Build history of the part. All positions in model axes, mm. A direction names the side the tool comes from. Give positions to 0.01 mm unless a question says otherwise; leave off trailing zeros. Loops run counter-clockwise (first coordinate to the right, second up) from the corner with the lowest first, then second, coordinate; pieces in that order, holes last. Notation, with made-up numbers: (-28.5, 54) -> (-3.5, 54) arc R9 cw to (-3.5, 65) -> close; hole circle Ø6 at (-29.5, 55.25). An arc over 180 degrees is marked (long way). Answer as a JSON object with one key per item and string values. Group by question number.
Q1. Wall check: probe 1 along X at (y, z) = (15.5, -38); probe 2 along Y at (x, z) = (0, -97) (3 decimals); probe 3 along X at (y, z) = (-5, -59). Give the ranges that are in metal, low to high. Write a range as from..to.
Q2. Band-saw the part on A-A, the plane x = 0. Write the cut outline in (y, z) (3 decimals), plus the area to 3 significant figures.
Q3. Two-plate mould, pull along Y, no slides. Class faces 4 (the flat face through (3, 3, 0)), 5 (the flat face through (0, -7.685, -148)), 6 (the cylindrical face through (-0.74, -3.32, -147.9)): pulls with the +Y half, pulls with the -Y half, needs draft (parallel to the pull), parting line crosses it, or undercut.
Q4. Band-saw the part on C-C, the plane z = -227. Count the separate pieces of the cut face and the enclosed holes in it, plus the area to 3 significant figures.
Q5. Drop flat-ended pins along their axis: pin 1 (7.5 mm diameter, centred on y = -1, z = -130.5, fed in from +X); pin 2 (0.7 mm diameter, centred on x = 18, z = -213, fed in from +Y); pin 3 (3.5 mm diameter, centred on x = 1, z = -81.5, fed in from +Y) (3 decimals). Give the stop position or say it passes through.
Q6. Tool access for faces 1 (the flat face through (0, 7.685, -148)), 2 (the flat face through (7.685, 0, -148)), 3 (the flat face through (-11.931, -14, -148)): list every direction of +Z, -Z, +X, -X, +Y, -Y with a clear straight run to the whole face (end or side of a thin tool).
Q7. Band-saw the part on B-B, the plane y = 0. Write the cut outline in (x, z) (3 decimals), plus the area to 3 significant figures.
from build123d import *

# Parameters (mm, degrees)
SKETCH1_R      = 3.4
EXTRUDE1_DEPTH = 300


with BuildPart() as part:
    # Sketch1 → Extrude1 (new body)
    with BuildSketch(Plane.XY):
        with BuildLine():
            Line((3.546734719, 7.685), (-3.215668941, 7.685))
            ThreePointArc((-3.215668941, 7.685), (-5.12166397, 8.084192802), (-6.707283616, 9.214671586))
            Line((-6.707283616, 9.214671586), (-9.994083925, 12.501471895))
            ThreePointArc((-9.994083925, 12.501471895), (-10.186794901, 12.789884252), (-10.254465997, 13.130089823))
            Line((-10.254465997, 13.130089823), (-10.254465997, 15.428464473))
            ThreePointArc((-10.254465997, 15.428464473), (-9.882491609, 16.326490085), (-8.984465997, 16.698464473))
            Line((-8.984465997, 16.698464473), (-6.775217878, 16.698464473))
            Line((-6.775217878, 16.698464473), (-6.775217878, 15.936))
            Line((-6.775217878, 15.936), (-5.6348, 15.936))
            ThreePointArc((-5.6348, 15.936), (-4.521248241, 16.397248241), (-4.06, 17.5108))
            Line((-4.06, 17.5108), (-4.06, 18.4252))
            ThreePointArc((-4.06, 18.4252), (-4.521248241, 19.538751759), (-5.6348, 20))
            Line((-5.6348, 20), (-13.0175, 20))
            Line((-13.0175, 20), (-16.825, 20))
            ThreePointArc((-16.825, 20), (-19.07006403, 19.07006403), (-20, 16.825))
            Line((-20, 16.825), (-20, -16.825))
            ThreePointArc((-20, -16.825), (-19.07006403, -19.07006403), (-16.825, -20))
            Line((-16.825, -20), (-13.0175, -20))
            Line((-13.0175, -20), (-5.6348, -20))
            ThreePointArc((-5.6348, -20), (-4.521248241, -19.538751759), (-4.06, -18.4252))
            Line((-4.06, -18.4252), (-4.06, -17.5108))
            ThreePointArc((-4.06, -17.5108), (-4.521248241, -16.397248241), (-5.6348, -15.936))
            Line((-5.6348, -15.936), (-6.775217878, -15.936))
            Line((-6.775217878, -15.936), (-6.775217878, -16.698464473))
            Line((-6.775217878, -16.698464473), (-8.984465997, -16.698464473))
            ThreePointArc((-8.984465997, -16.698464473), (-9.882491609, -16.326490085), (-10.254465997, -15.428464473))
            Line((-10.254465997, -15.428464473), (-10.254465997, -13.130554296))
            ThreePointArc((-10.254465997, -13.130554296), (-10.186794901, -12.790348725), (-9.994083925, -12.501936368))
            Line((-9.994083925, -12.501936368), (-6.707283616, -9.215136058))
            ThreePointArc((-6.707283616, -9.215136058), (-5.121525017, -8.084319577), (-3.21524064, -7.685))
            Line((-3.21524064, -7.685), (3.384844934, -7.685))
            ThreePointArc((3.384844934, -7.685), (5.234788394, -8.060064667), (6.792572846, -9.126025224))
            Line((6.792572846, -9.126025224), (9.994035567, -12.327487945))
            ThreePointArc((9.994035567, -12.327487945), (10.186746543, -12.615900302), (10.254417639, -12.956105874))
            Line((10.254417639, -12.956105874), (10.254417639, -15.439547173))
            ThreePointArc((10.254417639, -15.439547173), (9.878564697, -16.3303999), (8.984465997, -16.698464473))
            Line((8.984465997, -16.698464473), (6.775217878, -16.698464473))
            Line((6.775217878, -16.698464473), (6.775217878, -15.936))
            Line((6.775217878, -15.936), (5.6348, -15.936))
            ThreePointArc((5.6348, -15.936), (4.521248241, -16.397248241), (4.06, -17.5108))
            Line((4.06, -17.5108), (4.06, -18.4252))
            ThreePointArc((4.06, -18.4252), (4.521248241, -19.538751759), (5.6348, -20))
            Line((5.6348, -20), (13.34169248, -20))
            Line((13.34169248, -20), (17.15169248, -20))
            ThreePointArc((17.15169248, -20), (19.188402964, -18.962027535), (20, -16.825))
            Line((20, -16.825), (20, -13.015))
            Line((20, -13.015), (20, -5.5728))
            ThreePointArc((20, -5.5728), (19.517832289, -4.499539536), (18.426420946, -4.06))
            Line((18.426420946, -4.06), (17.5148, -4.06))
            ThreePointArc((17.5148, -4.06), (16.401248241, -4.521248241), (15.94, -5.6348))
            Line((15.94, -5.6348), (15.94, -6.775217878))
            Line((15.94, -6.775217878), (16.702464473, -6.775217878))
            Line((16.702464473, -6.775217878), (16.702464473, -8.984465997))
            ThreePointArc((16.702464473, -8.984465997), (16.363032482, -9.986041481), (15.382992443, -10.383394031))
            Line((15.382992443, -10.383394031), (13.085082266, -10.383394031))
            ThreePointArc((13.085082266, -10.383394031), (12.744876695, -10.315722936), (12.456464338, -10.12301196))
            Line((12.456464338, -10.12301196), (9.169664028, -6.83621165))
            ThreePointArc((9.169664028, -6.83621165), (8.107276575, -5.34917353), (7.685, -3.571075679))
            Line((7.685, -3.571075679), (7.685, 3.191327981))
            ThreePointArc((7.685, 3.191327981), (7.983205038, 5.049694415), (8.979790179, 6.646337802))
            Line((8.979790179, 6.646337802), (12.266590489, 9.933138111))
            ThreePointArc((12.266590489, 9.933138111), (12.592412986, 10.262627227), (13.039781689, 10.383394031))
            Line((13.039781689, 10.383394031), (15.37809843, 10.383394031))
            ThreePointArc((15.37809843, 10.383394031), (16.251511682, 10.035375209), (16.646241073, 9.182054333))
            Line((16.646241073, 9.182054333), (16.646241073, 6.972806215))
            Line((16.646241073, 6.972806215), (15.94, 6.972806215))
            Line((15.94, 6.972806215), (15.94, 5.832388337))
            ThreePointArc((15.94, 5.832388337), (16.321009151, 4.593446811), (17.502355238, 4.06))
            Line((17.502355238, 4.06), (18.4252, 4.06))
            ThreePointArc((18.4252, 4.06), (19.538751759, 4.521248241), (20, 5.6348))
            Line((20, 5.6348), (20, 13.01422635))
            Line((20, 13.01422635), (20, 16.82422635))
            ThreePointArc((20, 16.82422635), (19.070337634, 19.069790487), (16.825000094, 20))
            Line((16.825000094, 20), (13.290515583, 20))
            Line((13.290515583, 20), (5.6348, 20))
            ThreePointArc((5.6348, 20), (4.521248241, 19.538751759), (4.06, 18.4252))
            Line((4.06, 18.4252), (4.06, 17.5108))
            ThreePointArc((4.06, 17.5108), (4.521248241, 16.397248241), (5.6348, 15.936))
            Line((5.6348, 15.936), (6.775217878, 15.936))
            Line((6.775217878, 15.936), (6.775217878, 16.698464473))
            Line((6.775217878, 16.698464473), (8.984465997, 16.698464473))
            ThreePointArc((8.984465997, 16.698464473), (9.921702832, 16.349296475), (10.315534003, 15.429933551))
            Line((10.315534003, 15.429933551), (10.315534003, 13.130863473))
            ThreePointArc((10.315534003, 13.130863473), (10.284388293, 12.763467996), (10.106856362, 12.44030874))
            Line((10.106856362, 12.44030874), (6.825600792, 9.15905317))
            ThreePointArc((6.825600792, 9.15905317), (5.331011713, 8.099837434), (3.546734719, 7.685))
        make_face()
        Circle(SKETCH1_R, mode=Mode.SUBTRACT)
        with BuildLine():
            Line((11.904417639, 17.715), (11.904417639, 13.303394031))
            ThreePointArc((11.904417639, 13.303394031), (12.276392027, 12.405368419), (13.174417639, 12.033394031))
            Line((13.174417639, 12.033394031), (17.715, 12.033394031))
            ThreePointArc((17.715, 12.033394031), (18.164012806, 12.219381225), (18.35, 12.668394031))
            Line((18.35, 12.668394031), (18.35, 15.556))
            ThreePointArc((18.35, 15.556), (17.531656347, 17.531656347), (15.556, 18.35))
            Line((15.556, 18.35), (12.539417639, 18.35))
            ThreePointArc((12.539417639, 18.35), (12.090404833, 18.164012806), (11.904417639, 17.715))
        make_face(mode=Mode.SUBTRACT)
        with BuildLine():
            Line((-12.566039342, -18.35), (-15.556000403, -18.35))
            ThreePointArc((-15.556000403, -18.35), (-17.531126348, -17.532186606), (-18.35, -15.5575))
            Line((-18.35, -15.5575), (-18.35, 15.5575))
            ThreePointArc((-18.35, 15.5575), (-17.531126348, 17.532186606), (-15.556000403, 18.35))
            Line((-15.556000403, 18.35), (-12.566039304, 18.35))
            ThreePointArc((-12.566039304, 18.35), (-12.11943409, 18.166407557), (-11.931075623, 17.721791441))
            Line((-11.931075623, 17.721791441), (-11.931075623, 10.955502483))
            ThreePointArc((-11.931075623, 10.955502483), (-11.717102891, 9.676453683), (-11.00956403, 8.589651528))
            Line((-11.00956403, 8.589651528), (-9.076184211, 6.656271709))
            ThreePointArc((-9.076184211, 6.656271709), (-8.046556996, 5.115325687), (-7.685, 3.29765592))
            Line((-7.685, 3.29765592), (-7.685, -3.46474774))
            ThreePointArc((-7.685, -3.46474774), (-8.065971567, -5.27844769), (-9.112016323, -6.808296445))
            Line((-9.112016323, -6.808296445), (-11.065958077, -8.720893286))
            ThreePointArc((-11.065958077, -8.720893286), (-11.717420577, -9.753448518), (-11.931075623, -10.95549894))
            Line((-11.931075623, -10.95549894), (-11.931075623, -17.721787898))
            ThreePointArc((-11.931075623, -17.721787898), (-12.119432868, -18.166406311), (-12.566039342, -18.35))
        make_face(mode=Mode.SUBTRACT)
        with BuildLine():
            Line((15.556, -18.35), (12.539417639, -18.35))
            ThreePointArc((12.539417639, -18.35), (12.090404833, -18.164012806), (11.904417639, -17.715))
            Line((11.904417639, -17.715), (11.904417639, -13.303394031))
            ThreePointArc((11.904417639, -13.303394031), (12.276392027, -12.405368419), (13.174417639, -12.033394031))
            Line((13.174417639, -12.033394031), (17.715, -12.033394031))
            ThreePointArc((17.715, -12.033394031), (18.164012806, -12.219381225), (18.35, -12.668394031))
            Line((18.35, -12.668394031), (18.35, -15.556))
            ThreePointArc((18.35, -15.556), (17.531656347, -17.531656347), (15.556, -18.35))
        make_face(mode=Mode.SUBTRACT)
    extrude(amount=-EXTRUDE1_DEPTH)


solid = part.part
Worked answers:
{
 "1": {"probe 1": "-20..-18.35, -11.93..-10.25, 10.31..11.9, 18.35..20", "probe 2": "-7.685..-3.4, 3.4..7.685", "probe 3": "-20..-18.35, -7.96..7.96, 16.07..19.87"},
 "2": {"outline": "(-7.685, -300) -> (-3.4, -300) -> (-3.4, 0) -> (-7.685, 0) -> close; (3.4, -300) -> (7.685, -300) -> (7.685, 0) -> (3.4, 0) -> close", "area": "2,570 mm2"},
 "3": {"face 4": "needs draft", "face 5": "pulls with the -Y half", "face 6": "undercut"},
 "4": {"separate pieces": "1", "enclosed holes": "4", "area": "632 mm2"},
 "5": {"pin 1": "x = 19.73", "pin 2": "y = 19.89", "pin 3": "y = 7.685"},
 "6": {"face 1": "+Z, -Z, +Y", "face 2": "+Z, -Z, +X", "face 3": "+Z, -Z"},
 "7": {"outline": "(-20, -300) -> (-18.35, -300) -> (-18.35, 0) -> (-20, 0) -> close; (-7.685, -300) -> (-3.4, -300) -> (-3.4, 0) -> (-7.685, 0) -> close; (3.4, -300) -> (7.685, -300) -> (7.685, 0) -> (3.4, 0) -> close", "area": "3,070 mm2"}
}
